Could you check a few things on this drawing? It's one solid part, dimensions in mm from its lowest x, y, z. A direction names the side the tool comes from. Give positions to 0.01 mm unless a question says otherwise; leave off trailing zeros. Loops run counter-clockwise (first coordinate to the right, second up) from the corner with the lowest first, then second, coordinate; pieces in that order, holes last. Notation, with made-up numbers: M 21,81.5 L 64,81.5 A16 cw 64,86.5 Z; hole C 52,-11.75 d8. An arc over 180 degrees is marked long. Answer in a Markdown table with one row per item. Add a question column.
1. If we section it at D-D on z = 23: List the corners of the cut face in (x, y) for me, then the cut area to 3 significant figures.
2. If we section it at B-B on x = 57: List the corners of the cut face in (y, z) for me.
3. If we section it at A-A on z = 37: List the corners of the cut face in (x, y) for me.
4. I need wall thicknesses on line 1 along X through (y, z) = (39, 15); line 2 along X through (y, z) = (24, 47); line 3 along Y through (x, z) = (15, 36). Which ranges of each line are inside material? Lowest first, please. Write a range as from..to.
5. If we section it at C-C on y = 64: List the corners of the cut face in (x, z) for me.
6. Which directions (+Z, -Z, +X, -X, +Y, -Y) give clear straight access to the entire face, cutting with the end or side of a thin tool? Please do the marked faces 1, 2 and 3.
7. I'm going to push flat-ended pins straight in: pin 1 Ø8 at (x, z) = (29.5, 58) entering from -Y; pin 2 Ø10 at (x, z) = (19.5, 51.5) entering from -Y; pin 3 Ø2.5 at (x, y) = (3.5, 35.5) entering from -Z; pin 4 Ø8 at (x, y) = (38.5, 31) entering from -Z. Where does each tip first touch, or does it pass through?
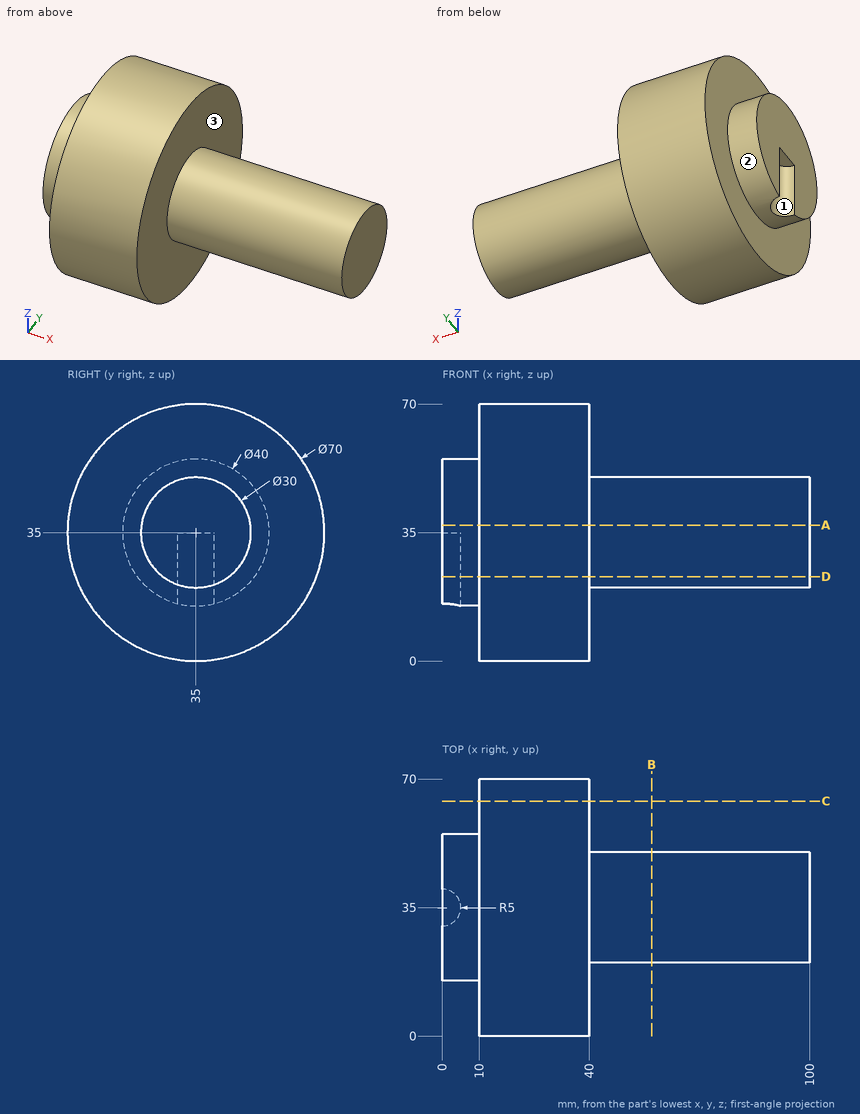
Results:
| question | item | result |
|---|---|---|
| 1 | outline | M 0,19 L 10,19 L 10,2.12 L 40,2.12 L 40,26 L 100,26 L 100,44 L 40,44 L 40,67.88 L 10,67.88 L 10,51 L 0,51 L 0,40 A5 cw 0,30 Z |
| 1 | area | 3,330 mm2 |
| 2 | outline | C 35,35 d30 |
| 3 | outline | M 0,15.1 L 10,15.1 L 10,0.06 L 40,0.06 L 40,20.13 L 100,20.13 L 100,49.87 L 40,49.87 L 40,69.94 L 10,69.94 L 10,54.9 L 0,54.9 Z |
| 4 | line 1 | 10..40 |
| 4 | line 2 | 0..40 |
| 4 | line 3 | 0.01..69.99 |
| 5 | outline | M 10,15.4 L 40,15.4 L 40,54.6 L 10,54.6 Z |
| 6 | face 1 | -Z, -X |
| 6 | face 2 | -X |
| 6 | face 3 | +X |
| 7 | pin 1 | y = 5.61 |
| 7 | pin 2 | y = 1.94 |
| 7 | pin 3 | z = 35 |
| 7 | pin 4 | z = 0 |
